```python
from build123d import *

# Parameters (mm, degrees)
SKETCH1_W           = 71.12
SKETCH1_H           = 71.12
BOSS_EXTRUDE1_DEPTH = 2.54
SKETCH2_R           = 15.24
CUT_EXTRUDE1_DEPTH  = 15.748
SKETCH4_R           = 1.905
CUT_EXTRUDE2_DEPTH  = 15.748


with BuildPart() as part:
    # Sketch1 → Boss-Extrude1 (new body)
    with BuildSketch(Plane(origin=(0, 0, 0), x_dir=(1, 0, 0), z_dir=(0, 1, 0))):
        with Locations((10.146850495, 4.656355231)):
            Rectangle(SKETCH1_W, SKETCH1_H)
    extrude(amount=-BOSS_EXTRUDE1_DEPTH)

    # Sketch2 → Cut-Extrude1 (cut)
    with BuildSketch(Plane(origin=(0, 0, 0), x_dir=(1, 0, 0), z_dir=(0, 1, 0))):
        with Locations(Location((10.146850495, 23.706355231, 0), (0, 0, 270))):
            Circle(SKETCH2_R)
    extrude(amount=-CUT_EXTRUDE1_DEPTH, mode=Mode.SUBTRACT)

    # Sketch4 → Cut-Extrude2 (cut)
    with BuildSketch(Plane(origin=(0, 0, 0), x_dir=(1, 0, 0), z_dir=(0, 1, 0))):
        with Locations(Location((10.146850495, 0.846355231, 0), (0, 0, 270))):
            Circle(SKETCH4_R)
    extrude(amount=-CUT_EXTRUDE2_DEPTH, mode=Mode.SUBTRACT)


solid = part.part
```
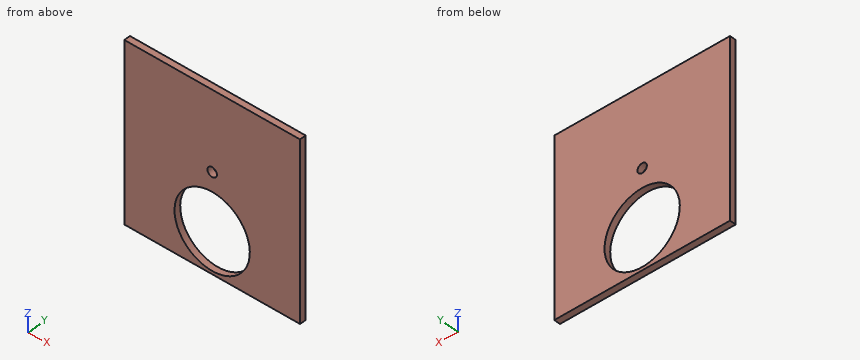
Could you check a few things on this model? Use its own coordinates, in mm. Coordinates: 2 decimals unless noted, no trailing zeros. Write each loop counter-clockwise with the first axis right and the second up, starting at its lowest first coordinate (ties: lowest second). Pieces come first, ordered by that corner, then holes. Notation, with made-up numbers: (6, 18.25) -> (38, 18.25) arc R29 ccw to (38, 39.25) -> close; hole circle Ø1 at (9.25, -39). An arc over 180 degrees is marked (long way). Return JSON: item names as keys, results as strings.
(1) I'm going to push a flat-ended pin straight in: pin 1 (2.5 mm diameter, centred on x = 10.15, z = -0.85, fed in from -Y). Where does the tip first touch, or does it pass through?
Numbers:
{"pin 1": "passes through"}
(2) Imagine slicing it at B-B, the plane z = -19. Please give me the cut outline in (x, y), then the cut area to 3 significant figures.
Numbers:
{"outline": "(-25.41, -2.54) -> (-4.35, -2.54) -> (-4.35, 0) -> (-25.41, 0) -> close; (24.64, -2.54) -> (45.71, -2.54) -> (45.71, 0) -> (24.64, 0) -> close", "area": "107 mm2"}
(3) Imagine slicing it at C-C, the plane y = -1.35. Please give me the cut outline in (x, z) (3 decimals).
Numbers:
{"outline": "(-25.413, -40.216) -> (45.707, -40.216) -> (45.707, 30.904) -> (-25.413, 30.904) -> close; hole circle Ø30.48 at (10.147, -23.706); hole circle Ø3.81 at (10.147, -0.846)"}
(4) Imagine slicing it at A-A, the plane x = 23. Please give me the cut outline in (y, z).
Numbers:
{"outline": "(-2.54, -40.22) -> (0, -40.22) -> (0, -31.9) -> (-2.54, -31.9) -> close; (-2.54, -15.52) -> (0, -15.52) -> (0, 30.9) -> (-2.54, 30.9) -> close"}
(5) I need wall thicknesses on L1, parallel to Z at x = 11, y = -1.3; L2, parallel to X at y = -0.15, z = -11; L3, parallel to Z at x = 21, y = -0.6. Which ranges of each line are inside material? Lowest first, please.
Numbers:
{"L1": "z = -40.22 to -38.92, -8.49 to -2.55, 0.86 to 30.9", "L2": "x = -25.41 to 1.73, 18.56 to 45.71", "L3": "z = -40.22 to -34.41, -13.01 to 30.9"}
